```python
from build123d import *

# Parameters (mm, degrees)
SKETCH_1_W          = 40
SKETCH_1_H          = 30
EXTRUDE_1_DEPTH     = 70
SKETCH_2_W          = 26
SKETCH_2_H          = 14
CUT_EXTRUDE_1_DEPTH = 65
SKETCH_3_W          = 5.2
SKETCH_3_H          = 5
CUT_EXTRUDE_2_DEPTH = 10
SKETCH_4_W          = 5.2
SKETCH_4_H          = 5
CUT_EXTRUDE_3_DEPTH = 10


with BuildPart() as part:
    # ｽｹｯﾁ1 → ﾎﾞｽ - 押し出し1 (new body)
    with BuildSketch(Plane.XY):
        Rectangle(SKETCH_1_W, SKETCH_1_H)
    extrude(amount=EXTRUDE_1_DEPTH)

    # ｽｹｯﾁ2 → ｶｯﾄ - 押し出し1 (cut)
    with BuildSketch(Plane(origin=(0, 0, 0), x_dir=(-1, 0, 0), z_dir=(0, 0, -1))):
        Rectangle(SKETCH_2_W, SKETCH_2_H)
    extrude(amount=-CUT_EXTRUDE_1_DEPTH, mode=Mode.SUBTRACT)

    # ｽｹｯﾁ3 → ｶｯﾄ - 押し出し2 (cut)
    with BuildSketch(Plane(origin=(0, 7, 0), x_dir=(-1, 0, 0), z_dir=(0, -1, 0))):
        with Locations((0, -2.5)):
            Rectangle(SKETCH_3_W, SKETCH_3_H)
    extrude(amount=-CUT_EXTRUDE_2_DEPTH, mode=Mode.SUBTRACT)

    # ｽｹｯﾁ4 → ｶｯﾄ - 押し出し3 (cut)
    with BuildSketch(Plane(origin=(0, -7, 0), x_dir=(1, 0, 0), z_dir=(0, 1, 0))):
        with Locations((0, -2.5)):
            Rectangle(SKETCH_4_W, SKETCH_4_H)
    extrude(amount=-CUT_EXTRUDE_3_DEPTH, mode=Mode.SUBTRACT)

    # Surface Cut 1
    split(bisect_by=Plane(origin=(0, 0, 0), x_dir=(-1, 0, 0), z_dir=(0, -1, 0)), keep=Keep.TOP)


solid = part.part
```
Here's how the part is built. I have some questions about the finished solid (model axes, mm). A direction names the side the tool comes from. Coordinates: 2 decimals unless noted, no trailing zeros. Loops run counter-clockwise (first coordinate to the right, second up) from the corner with the lowest first, then second, coordinate; pieces in that order, holes last. Notation, with made-up numbers: (12, 51) - (62, 51) arc R14 cw to (62, 62) - close; hole circle Ø7 at (-28, 10.25). An arc over 180 degrees is marked (long way). Return JSON: item names as keys, results as strings. Group by question number.
Item 1: If we section it at A-A on x = 12: Write out the boundary of the cut face in (y, z), and give its area (3 significant figures).
Item 2: If we section it at C-C on y = -1.75: Write out the boundary of the cut face in (x, z), and give its area (3 significant figures).
Item 3: Will these pins go through, and if not, where does the flat tip stop? P1, Ø2.5, axis at x = -0.5, y = -11.5, coming from the -Z side; P2, Ø5.5, axis at x = 2.5, y = -3, coming from the -Z side.
Item 4: On a 3-axis mill with a long thin cutter (end or side, diameter ignored), from which of +Z, -Z, +X, -X, +Y, -Y can I reach the whole of each face in a straight line? I mean faces 1 (the face through (13, -4, 32)), 2 (the face through (0, -15, 35)), 3 (the face through (-2.6, -11, 3)). Say none if no direction works.
Item 5: If we section it at B-B on z = 25: Write out the boundary of the cut face in (x, y), and give its area (3 significant figures).
Item 6: I need wall thicknesses on line 1 (X direction, y = -14, z = 4); line 2 (X direction, y = -1.5, z = 11.5); line 3 (Y direction, x = -6, z = 36.5). Which ranges of each line are inside material? Lowest first, please. Write a range as from..to.
Item 7: We'd pull the mould along X, two halves only. Please class faces 4 (the face through (0, -11, 5)), 5 (the face through (0, -7, 32)), 6 (the face through (-13, -9, 0)), 7 (the face through (-20, -8, 35)): +X half, -X half, draft (parallel to the pull), parting line (faces both ways), or undercut.
Calculated:
{
 "1": {"outline": "(-15, 0) - (-7, 0) - (-7, 65) - (0, 65) - (0, 70) - (-15, 70) - close", "area": "595 mm^2"},
 "2": {"outline": "(-20, 0) - (-13, 0) - (-13, 65) - (13, 65) - (13, 0) - (20, 0) - (20, 70) - (-20, 70) - close", "area": "1,110 mm^2"},
 "3": {"P1": "stops at z = 5", "P2": "stops at z = 65"},
 "4": {"face 1": "-Z, +Y", "face 2": "+Z, -Z, +X, -X, -Y", "face 3": "-Z, +Y, -Y"},
 "5": {"outline": "(-20, -15) - (20, -15) - (20, 0) - (13, 0) - (13, -7) - (-13, -7) - (-13, 0) - (-20, 0) - close", "area": "418 mm^2"},
 "6": {"line 1": "x = -20..-2.6, 2.6..20", "line 2": "x = -20..-13, 13..20", "line 3": "y = -15..-7"},
 "7": {"face 4": "undercut", "face 5": "undercut", "face 6": "draft", "face 7": "-X half"}
}
